Input: dimensioned drawing with shaded views. Units: mm. Origin: part minimum x, y, z. Coordinates: 2 decimals unless noted, no trailing zeros. Loops run counter-clockwise (first coordinate to the right, second up) from the corner with the lowest first, then second, coordinate; pieces in that order, holes last.
(1) Section B-B, the plane z = 153. Return loops of the section in (x, y), then the cut area to 3 significant figures.
(2) Contact query for flat-ended pins moving along their axis: P1, Ø1.2, axis at y = 1.5, z = 2, coming from the -X side; P2, Ø2, axis at x = 1.5, y = 2, coming from the -Z side; P3, Ø1.8, axis at x = 5.7, z = 153, coming from the +Y side. Output: stop coordinate, or through.
(3) Section A-A, the plane x = 67.7. Return loops of the section in (y, z), then the cut area to 3 significant figures.
(4) Line query: L1, parallel to X at y = 1, z = 153; L2, parallel to Z at x = 67.7, y = 1.4. Output: solid intervals per line, ascending.
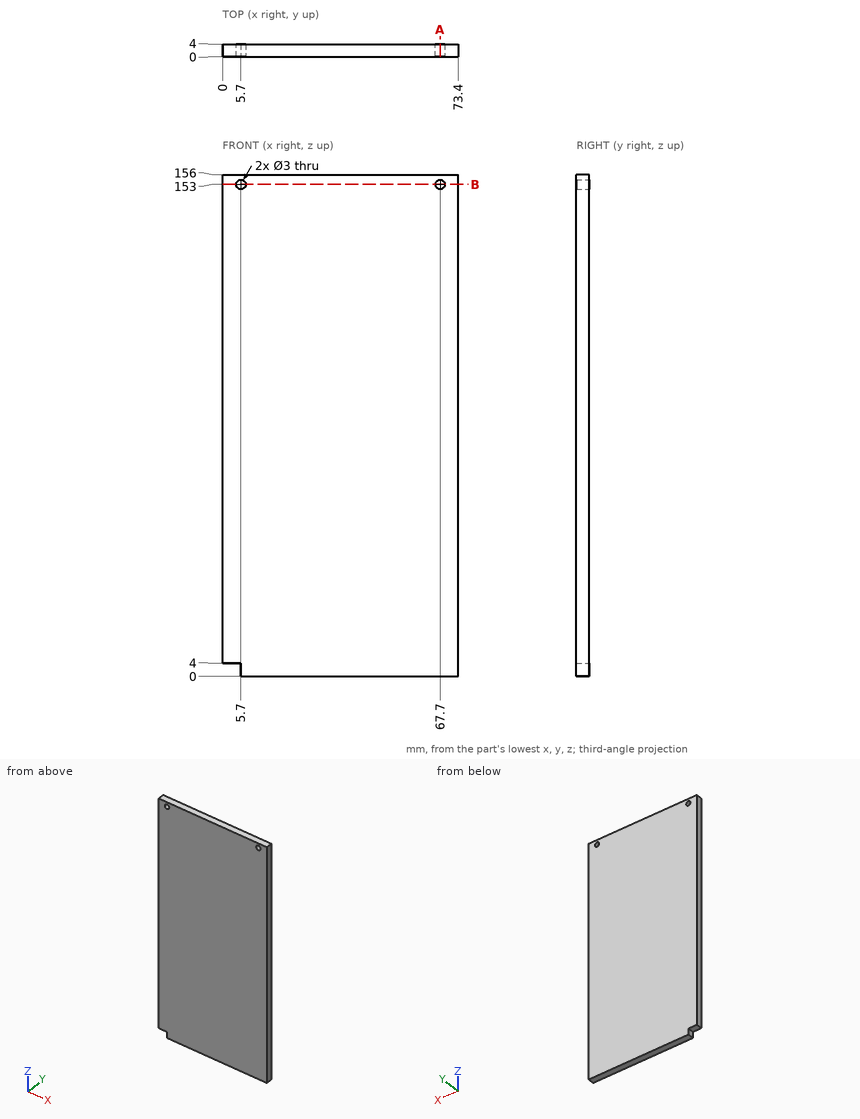
Report:
1. outline: (0, 0) - (4.2, 0) - (4.2, 4) - (0, 4) - close; (7.2, 0) - (66.2, 0) - (66.2, 4) - (7.2, 4) - close; (69.2, 0) - (73.4, 0) - (73.4, 4) - (69.2, 4) - close
1. area: 270 mm2
2. P1: stops at x = 5.7
2. P2: stops at z = 4
2. P3: passes through
3. outline: (0, 0) - (4, 0) - (4, 151.5) - (0, 151.5) - close; (0, 154.5) - (4, 154.5) - (4, 156) - (0, 156) - close
3. area: 612 mm2
4. L1: x = 0 to 4.2, 7.2 to 66.2, 69.2 to 73.4
4. L2: z = 0 to 151.5, 154.5 to 156
